Part print with two shaded views. Sizes in mm from the minimum x, y, z corner. A direction names the side the tool comes from. Round coordinates to 2 decimals unless told otherwise and drop trailing zeros. Write each loop counter-clockwise with the first axis right and the second up, starting at its lowest first coordinate (ties: lowest second). Pieces come first, ordered by that corner, then holes. Notation, with made-up numbers: (35, 85.5) -> (86, 85.5) arc R22 ccw to (86, 117.5) -> close; hole circle Ø10 at (30, -28). An arc over 180 degrees is marked (long way). Put each result on its own line as item: value. Start each with the question number.
1. Flat gauge pins, fed straight in: P1, Ø1.5, axis at x = 8.5, y = 14, coming from the +Z side; P2, Ø1.5, axis at y = 5, z = 26, coming from the +X side; P3, Ø1, axis at x = 6.5, z = 16.5, coming from the -Y side; P4, Ø1.2, axis at y = 28.5, z = 15.5, coming from the -X side. Where does each tip first touch, or does it go through?
2. Saw through at B-B on x = 15. List the corners of the cut face in (y, z).
3. Drill centre lines: line 1 (X direction, y = 11, z = 14.25); line 2 (Z direction, x = 7.5, y = 14.5); line 3 (Y direction, x = 35.5, z = 12.5). Where is each one in solid material? Low to high. Write a range as from..to.
4. 3-axis set-ups, long thin cutter, end or side, ignore diameter. For the marked faces 5, 6, 7, 8 and 9: which of +Z, -Z, +X, -X, +Y, -Y reach the whole face in a straight line?
5. Pull direction X, two halves, no side cores. Call the marked faces 1, 2, 3 and 4: pulls with the +X half, pulls with the -X half, needs draft (parallel to the pull), parting line crosses it, or undercut.
6. Saw through at D-D on z = 15.5. List the corners of the cut face in (x, y), and give its area (3 significant figures).
7. Saw through at A-A on y = 17. List the corners of the cut face in (x, z).
8. Saw through at C-C on y = 27. List the corners of the cut face in (x, z), and give its area (3 significant figures).
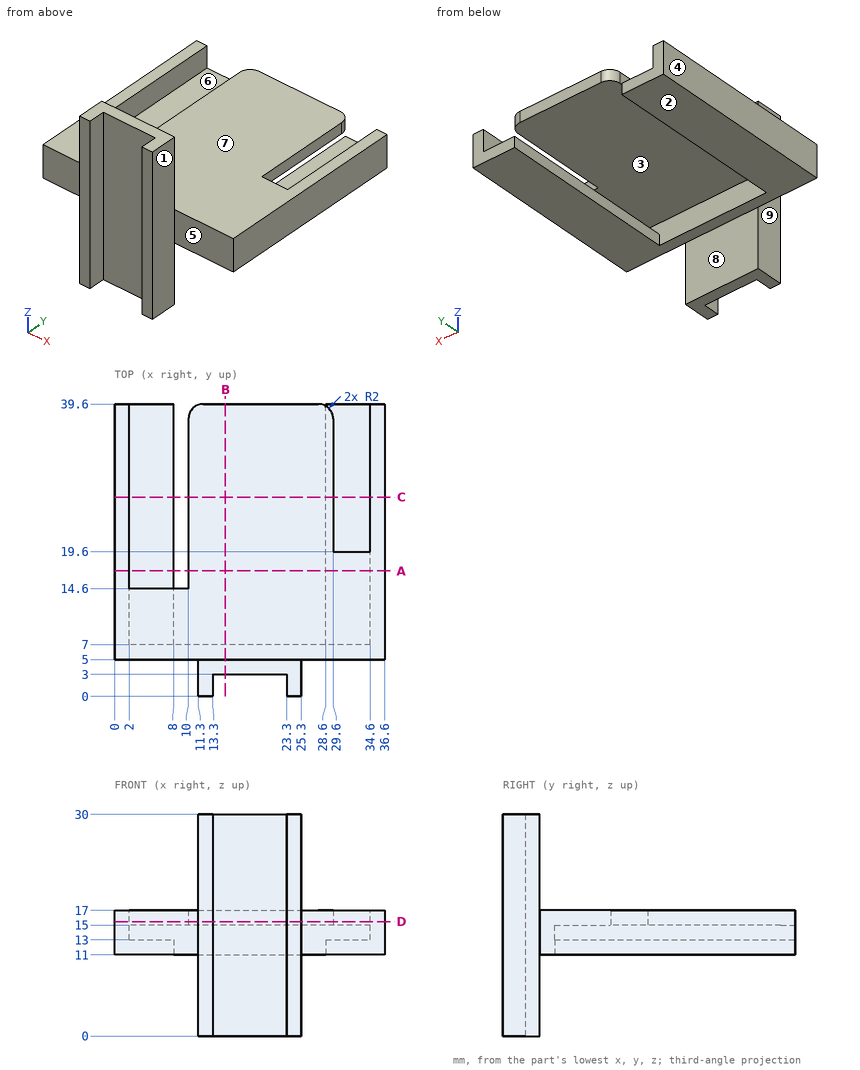
Return value:
1. P1: stops at z = 17
1. P2: stops at x = 25.3
1. P3: stops at y = 5
1. P4: stops at x = 0
2. outline: (3, 0) -> (5, 0) -> (5, 11) -> (7, 11) -> (7, 15) -> (39.6, 15) -> (39.6, 17) -> (5, 17) -> (5, 30) -> (3, 30) -> close
3. line 1: x = 0..2, 34.6..36.6
3. line 2: z = 11..13, 15..17
3. line 3: y = 5..39.6
4. face 5: +Z, -Z, +X, -Y
4. face 6: +Y
4. face 7: +Z, +X, -X, +Y
4. face 8: -Z, +X, -X, +Y
4. face 9: +Z, -Z, -X, -Y
5. face 1: pulls with the +X half
5. face 2: needs draft
5. face 3: undercut
5. face 4: pulls with the -X half
6. outline: (0, 5) -> (11.3, 5) -> (11.3, 0) -> (13.3, 0) -> (13.3, 3) -> (23.3, 3) -> (23.3, 0) -> (25.3, 0) -> (25.3, 5) -> (36.6, 5) -> (36.6, 39.6) -> (34.6, 39.6) -> (34.6, 19.6) -> (29.6, 19.6) -> (29.6, 37.6) arc R2 ccw to (27.6, 39.6) -> (12, 39.6) arc R2 ccw to (10, 37.6) -> (10, 14.6) -> (2, 14.6) -> (2, 39.6) -> (0, 39.6) -> close
6. area: 1,000 mm^2
7. outline: (0, 11) -> (8, 11) -> (8, 13) -> (2, 13) -> (2, 17) -> (0, 17) -> close; (10, 15) -> (34.6, 15) -> (34.6, 13) -> (28.6, 13) -> (28.6, 11) -> (36.6, 11) -> (36.6, 17) -> (10, 17) -> close
8. outline: (0, 11) -> (8, 11) -> (8, 13) -> (2, 13) -> (2, 17) -> (0, 17) -> close; (10, 15) -> (29.6, 15) -> (29.6, 17) -> (10, 17) -> close; (28.6, 11) -> (36.6, 11) -> (36.6, 17) -> (34.6, 17) -> (34.6, 13) -> (28.6, 13) -> close
8. area: 87.2 mm^2
